Check sheet for the drawn part. Datum: minimum x, y, z corner. Units: mm. A direction names the side the tool comes from. Round coordinates to 2 decimals unless told otherwise and drop trailing zeros. Loops run counter-clockwise (first coordinate to the right, second up) from the corner with the lowest first, then second, coordinate; pieces in that order, holes last. Notation, with made-up numbers: (76, 47) -> (103, 47) arc R26 cw to (103, 79) -> close; hole circle Ø11 at (22, 31.25). An arc over 180 degrees is marked (long way). Return JSON: item names as keys, results as strings.
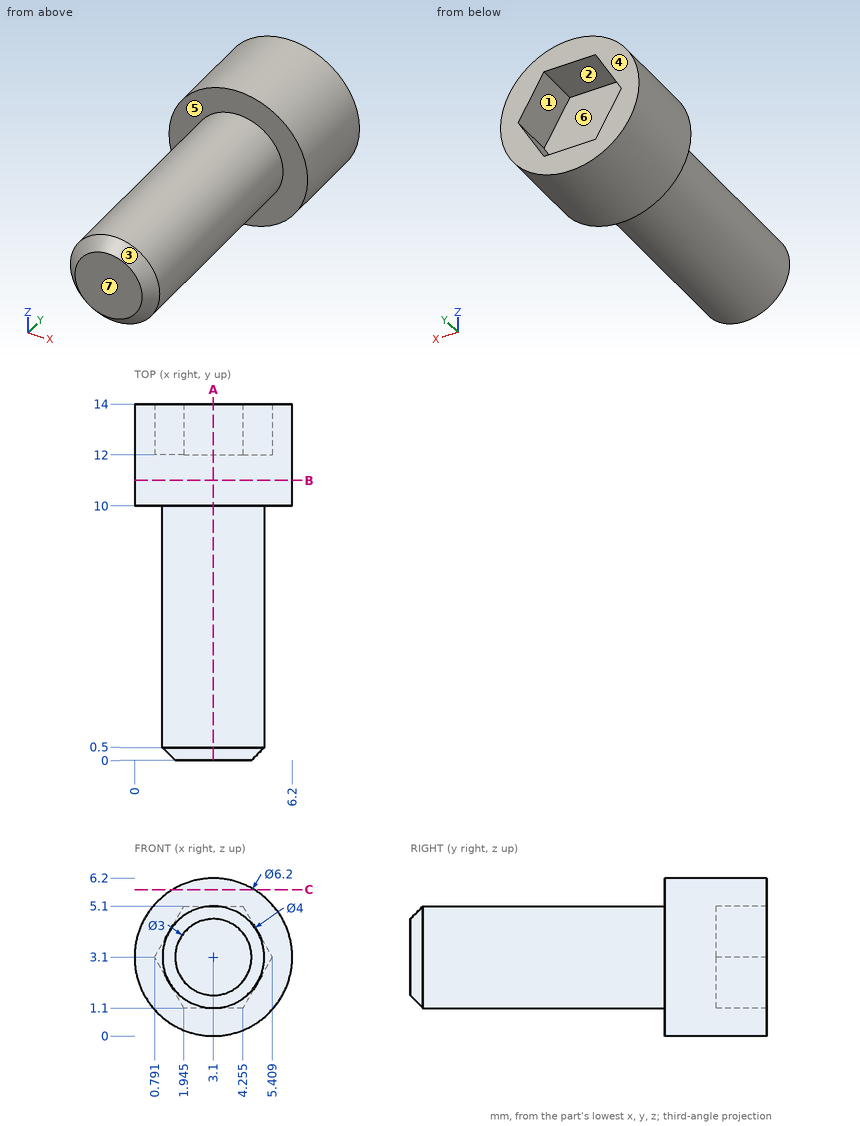
Q1. Section check C-C (z = 5.75). Record the boundary of the cut face in (x, y), then the cut area to 3 significant figures.
Results list:
{"outline": "(1.49, 10) -> (4.71, 10) -> (4.71, 14) -> (1.49, 14) -> close", "area": "12.9 mm^2"}
Q2. Draft check along Z on the marked faces 1, 2, 3 and 4. Enter one of: released by +Z, released by -Z, zero draft, split by the parting line, or undercut.
Results list:
{"face 1": "undercut", "face 2": "undercut", "face 3": "split by the parting line", "face 4": "zero draft"}
Q3. Section check B-B (y = 11). Record the boundary of the cut face in (x, z), then the cut area to 3 significant figures.
Results list:
{"outline": "circle Ø6.2 at (3.1, 3.1)", "area": "30.2 mm^2"}
Q4. Tool access check on the marked faces 5, 6 and 7. Record the directions out of +Z, -Z, +X, -X, +Y, -Y that give a thin tool (end or side, any length) a straight path to the whole face; none if there is none.
Results list:
{"face 5": "-Y", "face 6": "+Y", "face 7": "+Z, -Z, +X, -X, -Y"}
Q5. Section check A-A (x = 3.1). Record the boundary of the cut face in (y, z).
Results list:
{"outline": "(0, 1.6) -> (0.5, 1.1) -> (10, 1.1) -> (10, 0) -> (14, 0) -> (14, 1.1) -> (12, 1.1) -> (12, 5.1) -> (14, 5.1) -> (14, 6.2) -> (10, 6.2) -> (10, 5.1) -> (0.5, 5.1) -> (0, 4.6) -> close"}
Q6. Go/stop test with flat-tipped pins: pin 1 (2 mm diameter, centred on x = 4.5, y = 6.5, fed in from -Z); pin 2 (2 mm diameter, centred on y = 2, z = 3, fed in from +X); pin 3 (2 mm diameter, centred on x = 3, z = 3, fed in from +Y). Record where each tip stops, or that it passes through.
Results list:
{"pin 1": "z = 1.14", "pin 2": "x = 5.1", "pin 3": "y = 12"}
Q7. Material ranges on line 1 (X direction, y = 12.75, z = 2) (1 decimal); line 2 (Y direction, x = 5.5, z = 3.75); line 3 (Y direction, x = 2.75, z = 2), recorded low to high.
Results list:
{"line 1": "0.2 to 1.4, 4.8 to 6", "line 2": "10 to 14", "line 3": "0 to 12"}
